The drawing under review shows one solid part. Ordinate dimensions are in mm from its lowest x, y, z. A direction names the side the tool comes from. Coordinates: 2 decimals unless noted, no trailing zeros. Order: outer loops, then holes, each group sorted by start corner. A loop starts at its lowest first (then second) coordinate and runs counter-clockwise, first axis right, second up. Notation, with made-up numbers: (84, -3.5) -> (102, -3.5) arc R9 ccw to (102, 5.5) -> close; hole circle Ø10 at (18.5, 23.5). An arc over 180 degrees is marked (long way). Use a Markdown table: item, result. Add a question column.
Q1. Add section C-C (x = 4). State the section outline as (y, z) points (3 decimals), then the cut area to 3 significant figures.
Q2. Machinability: for the marked faces 4 and 5, which of the approach directions +Z, -Z, +X, -X, +Y, -Y give a long, thin tool a straight path to every point of the face, cutting with its end or side? Answer none if there is none.
Q3. The part is to be moulded in two halves that separate along X. For the marked faces 1, 2 and 3, say which applies: pulls with the +X half, pulls with the -X half, needs draft (parallel to the pull), parting line crosses it, or undercut.
Q4. Add section B-B (y = 8.5). State the section outline as (x, z) points, then the cut area to 3 significant figures.
Q5. Add section D-D (z = 4.5). State the section outline as (x, y) points.
Q6. Insertion check: pin 1 (2.5 mm diameter, centred on x = 4, y = 5.175, fed in from -Z); pin 2 (2.5 mm diameter, centred on y = 6.5, z = 5, fed in from -X); pin 3 (4 mm diameter, centred on x = 40, y = 9, fed in from -Z); pin 4 (1 mm diameter, centred on x = 57.5, z = 5, fed in from -Y) (3 decimals). Each pin has a flat end and moves straight along its axis. Give the tip position at first contact, or say it passes through.
Q7. Wall thickness on probe 1 along X at (y, z) = (5, 8.5); probe 2 along X at (y, z) = (7.5, 3.5); probe 3 along X at (y, z) = (7.25, 5.75): over which ranges is each line inside the solid? List them lowest first.
Q8. Add section A-A (z = 8). State the section outline as (x, y) points (3 decimals), then the cut area to 3 significant figures.
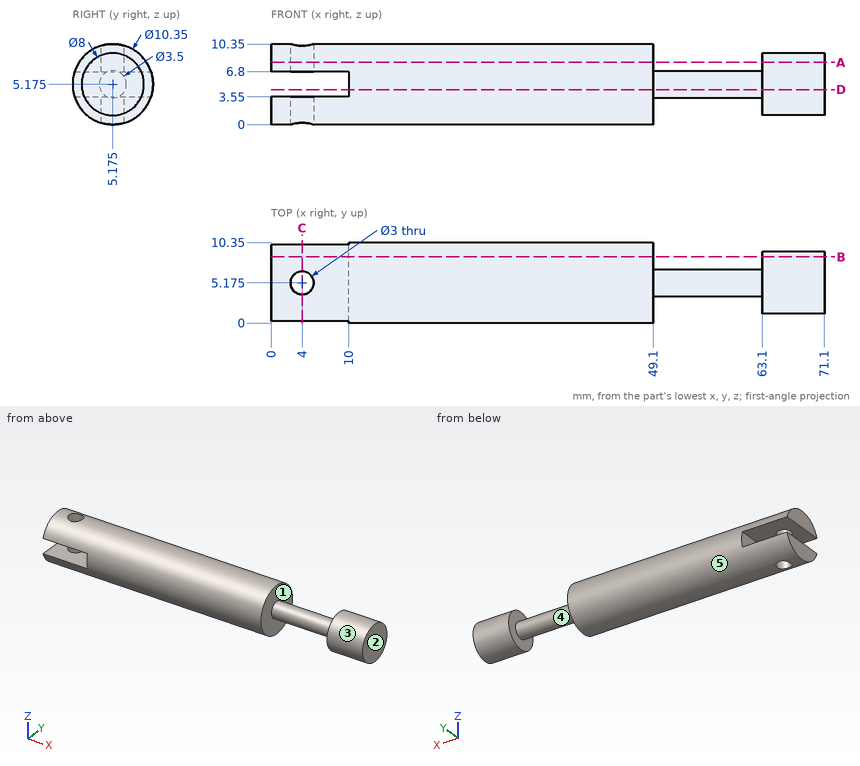
Established:
| question | item | result |
|---|---|---|
| 1 | outline | (0.262, 3.55) arc R5.175 ccw to (3.675, 0.222) -> (3.675, 3.55) -> close; (0.262, 6.8) -> (3.675, 6.8) -> (3.675, 10.128) arc R5.175 ccw to start; (6.675, 0.222) arc R5.175 ccw to (10.088, 3.55) -> (6.675, 3.55) -> close; (6.675, 6.8) -> (10.088, 6.8) arc R5.175 ccw to (6.675, 10.128) -> close |
| 1 | area | 30.2 mm^2 |
| 2 | face 4 | none |
| 2 | face 5 | +X, -X |
| 3 | face 1 | undercut |
| 3 | face 2 | pulls with the +X half |
| 3 | face 3 | needs draft |
| 4 | outline | (0, 1.21) -> (49.1, 1.21) -> (49.1, 9.14) -> (0, 9.14) -> (0, 6.8) -> (10, 6.8) -> (10, 3.55) -> (0, 3.55) -> close; (63.1, 2.95) -> (71.1, 2.95) -> (71.1, 7.4) -> (63.1, 7.4) -> close |
| 4 | area | 392 mm^2 |
| 5 | outline | (10, 0.04) -> (49.1, 0.04) -> (49.1, 3.56) -> (63.1, 3.56) -> (63.1, 1.23) -> (71.1, 1.23) -> (71.1, 9.12) -> (63.1, 9.12) -> (63.1, 6.79) -> (49.1, 6.79) -> (49.1, 10.31) -> (10, 10.31) -> close |
| 6 | pin 1 | through |
| 6 | pin 2 | x = 10 |
| 6 | pin 3 | z = 0.33 |
| 6 | pin 4 | y = 3.425 |
| 7 | probe 1 | 0 to 2.51, 5.49 to 49.1, 63.1 to 71.1 |
| 7 | probe 2 | 0 to 49.1, 63.1 to 71.1 |
| 7 | probe 3 | 10 to 49.1, 63.1 to 71.1 |
| 8 | outline | (0, 0.839) -> (49.1, 0.839) -> (49.1, 9.511) -> (0, 9.511) -> close; (63.1, 2.343) -> (71.1, 2.343) -> (71.1, 8.007) -> (63.1, 8.007) -> close; hole circle Ø3 at (4, 5.175) |
| 8 | area | 464 mm^2 |
